Build history of the part. All positions in model axes, mm. A direction names the side the tool comes from. Give positions to 0.01 mm unless a question says otherwise; leave off trailing zeros. Write each loop counter-clockwise with the first axis right and the second up, starting at its lowest first coordinate (ties: lowest second). Pieces come first, ordered by that corner, then holes. Notation, with made-up numbers: (-4, -26.75) -> (35, -26.75) arc R30 ccw to (35, -4.75) -> close; hole circle Ø3 at (19.5, 77.5). An arc over 180 degrees is marked (long way). Write item = value, one per line. Start each with the question number.
Q1. Mould opens along Y. For faces 4 (the face through (0, -1.587, 1)), 5 (the face through (0.133, 5.675, 24.775)), 6 (the face through (-5.056, -4.625, -45.971)), 7 (the face through (0, -7, -41.275)) say: pulls with the +Y half, pulls with the -Y half, needs draft (parallel to the pull), parting line crosses it, or undercut.
Q2. Saw through at B-B, the plane y = -11. List the corners of the cut face in (x, z) (1 decimal), then the cut area to 3 significant figures.
Q3. Drop flat-ended pins along their axis: P1, Ø2, axis at x = 5.5, z = 9, coming from the -Y side; P2, Ø4.5, axis at x = -3.175, y = -6.35, coming from the +Z side. Give the stop position or say it passes through.
Q4. Saw through at A-A, the plane x = -2.25. List the corners of the cut face in (y, z) (1 decimal).
Q5. Tool access for faces 1 (the face through (0, -7, 41.275)), 2 (the face through (0.133, 5.675, -19.675)), 3 (the face through (5.316, -4.329, 43.546)): list every direction of +Z, -Z, +X, -X, +Y, -Y with a clear straight run to the whole face (end or side of a thin tool).
Q6. Saw through at D-D, the plane z = -31. List the corners of the cut face in (x, y) (1 decimal).
Q7. Wall check: line 1 (Z direction, x = 4.5, y = -9.25) (3 decimals); line 2 (Y direction, x = 4.75, z = -22); line 3 (Z direction, x = -5.25, y = 5). Give the ranges that are in metal, low to high.
Q8. Saw through at C-C, the plane y = -7.25. List the corners of the cut face in (x, z) (1 decimal), then the cut area to 3 significant figures.
from build123d import *

# Parameters (mm, degrees)
SKETCH1_W                   = 19.05
SKETCH1_H                   = 25.4
EXTRUDE1_DEPTH              = 50.8
CUT_EXTRUDE1_REACH          = 21.05
SKETCH2_W                   = 82.55
SKETCH2_H                   = 11.1125
F_1_4_20_TAPPED_HOLE1_D     = 5.1054
F_1_4_20_TAPPED_HOLE1_DEPTH = 9.525
F_1_4_20_TAPPED_HOLE2_D     = 5.1054
F_1_4_20_TAPPED_HOLE2_DEPTH = 9.525
F_1_4_20_TAPPED_HOLE3_D     = 5.1054
F_1_4_20_TAPPED_HOLE3_DEPTH = 16.51
F_1_4_20_TAPPED_HOLE3_TIP   = 1.533816902
F_1_4_20_TAPPED_HOLE4_D     = 5.1054
F_1_4_20_TAPPED_HOLE4_DEPTH = 19.05


with BuildPart() as part:
    # Sketch1 → Extrude1 (new body, symmetric)
    with BuildSketch(Plane.XY):
        Rectangle(SKETCH1_W, SKETCH1_H)
    extrude(amount=EXTRUDE1_DEPTH, both=True)

    # Sketch2 → Cut-Extrude1 (cut, up to next)
    with BuildSketch(Plane(origin=(9.525, 0, 0), x_dir=(0, 0, -1), z_dir=(1, 0, 0)), mode=Mode.PRIVATE) as cut_extrude1_sk1:
        with Locations((0, -7.14375)):
            Rectangle(SKETCH2_W, SKETCH2_H)
    cut_extrude1_tool1 = extrude(cut_extrude1_sk1.sketch, amount=-CUT_EXTRUDE1_REACH, mode=Mode.PRIVATE) & part.part
    add(cut_extrude1_tool1.solids().sort_by_distance((9.525, -7.14375, 0))[0], mode=Mode.SUBTRACT)

    # 1/4-20 Tapped Hole1
    with Locations(Plane(origin=(0, 0, -50.8), x_dir=(-1, 0, 0), z_dir=(0, 0, -1))):
        with Locations((3.175, -6.35)):
            Hole(F_1_4_20_TAPPED_HOLE1_D / 2, depth=F_1_4_20_TAPPED_HOLE1_DEPTH)

    # 1/4-20 Tapped Hole2
    with Locations(Plane.XY.offset(50.8)):
        with Locations((-3.175, -6.35)):
            Hole(F_1_4_20_TAPPED_HOLE2_D / 2, depth=F_1_4_20_TAPPED_HOLE2_DEPTH)

    # 1/4-20 Tapped Hole3
    with Locations(Plane.XZ.offset(12.7)):
        with Locations((4.7625, 46.0375), (4.7625, -46.0375)):
            Hole(F_1_4_20_TAPPED_HOLE3_D / 2, depth=F_1_4_20_TAPPED_HOLE3_DEPTH)
            with Locations((0, 0, -(F_1_4_20_TAPPED_HOLE3_DEPTH + F_1_4_20_TAPPED_HOLE3_TIP / 2))):  # 118° drill point
                Cone(0, F_1_4_20_TAPPED_HOLE3_D / 2, F_1_4_20_TAPPED_HOLE3_TIP, mode=Mode.SUBTRACT)

    # 1/4-20 Tapped Hole4
    with Locations(Plane.ZY.offset(9.525)):
        with Locations((-22.225, 5.5626), (22.225, 5.5626)):
            Hole(F_1_4_20_TAPPED_HOLE4_D / 2, depth=F_1_4_20_TAPPED_HOLE4_DEPTH)


solid = part.part
Report:
q1.face_4 = pulls with the -Y half
q1.face_5 = undercut
q1.face_6 = undercut
q1.face_7 = needs draft
q2.outline = (-9.5, -50.8) -> (9.5, -50.8) -> (9.5, -41.3) -> (-9.5, -41.3) -> close; (-9.5, 41.3) -> (9.5, 41.3) -> (9.5, 50.8) -> (-9.5, 50.8) -> close; hole circle Ø5.1 at (4.8, -46); hole circle Ø5.1 at (4.8, 46)
q2.area = 322 mm2
q3.P1 = -1.59
q3.P2 = through
q4.outline = (-12.7, -50.8) -> (-8.7, -50.8) -> (-8.7, -41.3) -> (-12.7, -41.3) -> close; (-12.7, 41.3) -> (-8.7, 41.3) -> (-8.7, 50.8) -> (-12.7, 50.8) -> close; (-4, -50.8) -> (12.7, -50.8) -> (12.7, 50.8) -> (-4, 50.8) -> (-4, 41.3) -> (-1.6, 41.3) -> (-1.6, -41.3) -> (-4, -41.3) -> close; hole circle Ø5.1 at (5.6, -22.2); hole circle Ø5.1 at (5.6, 22.2)
q5.face_1 = +X, -X, -Y
q5.face_2 = +X, -X
q5.face_3 = -Y
q6.outline = (-9.5, -1.6) -> (9.5, -1.6) -> (9.5, 12.7) -> (-9.5, 12.7) -> close
q7.line_1 = -50.8 to -48.577, -43.498 to -41.275, 41.275 to 43.498, 48.577 to 50.8
q7.line_2 = -1.59 to 3.02, 8.11 to 12.7
q7.line_3 = -50.8 to -24.71, -19.74 to 19.74, 24.71 to 50.8
q8.outline = (-9.5, -50.8) -> (-5.6, -50.8) -> (-5.6, -41.3) -> (-9.5, -41.3) -> close; (-9.5, 41.3) -> (-5.6, 41.3) -> (-5.6, 50.8) -> (-9.5, 50.8) -> close; (-0.8, -50.8) -> (9.5, -50.8) -> (9.5, -41.3) -> (-0.8, -41.3) -> close; (-0.8, 41.3) -> (9.5, 41.3) -> (9.5, 50.8) -> (-0.8, 50.8) -> close; hole circle Ø5.1 at (4.8, -46); hole circle Ø5.1 at (4.8, 46)
q8.area = 231 mm2
